Could you check a few things on this drawing? It's one solid part, dimensions in mm from its lowest x, y, z. A direction names the side the tool comes from. Give positions to 0.01 mm unless a question says otherwise; leave off trailing zeros. Order: outer loops, then holes, each group sorted by start corner. A loop starts at its lowest first (then second) coordinate and runs counter-clockwise, first axis right, second up. Notation, with made-up numbers: (4, -38) -> (26, -38) arc R20 cw to (26, -30) -> close; hole circle Ø1 at (-20, -31.75). An arc over 180 degrees is marked (long way). Use one line per item in the form item = value. Start each with the question number.
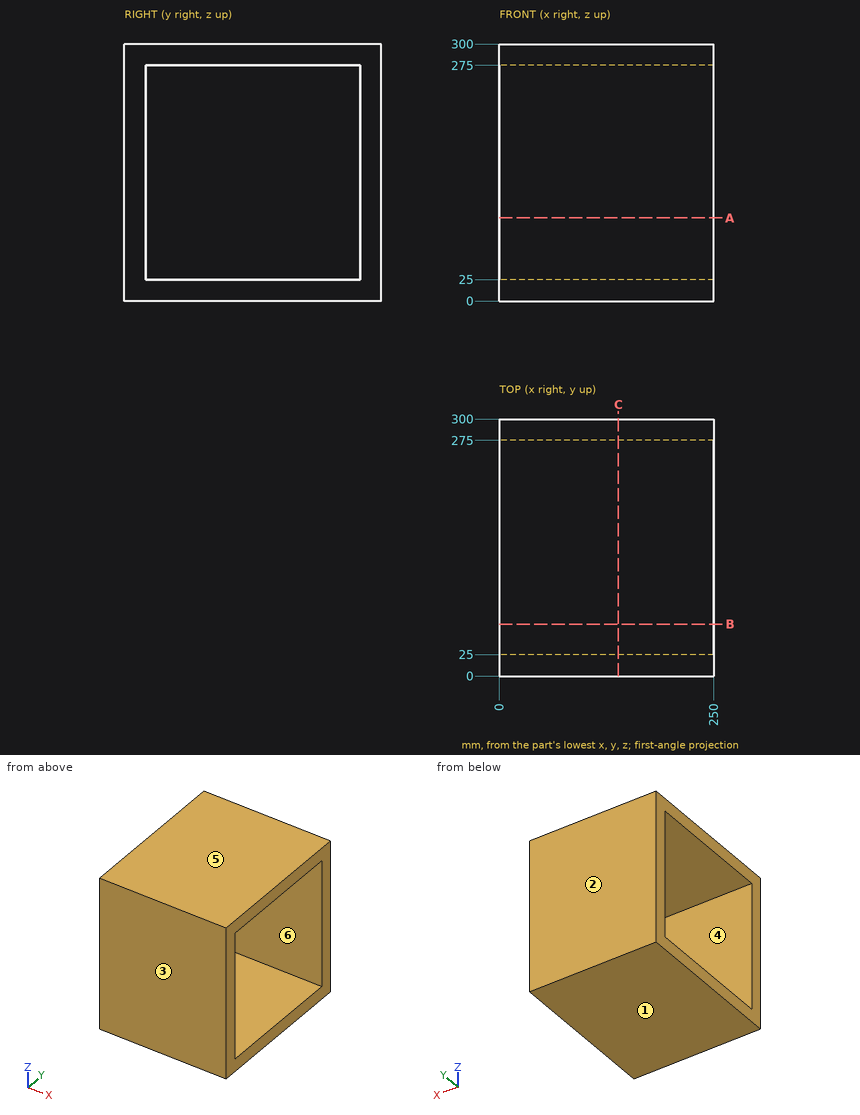
(1) Imagine slicing it at A-A (z = 97). Write out the boundary of the cut face in (x, y).
(2) Please list where this line runs through material, in increasing order: probe 1 along Z at (x, y) = (58.5, 240).
(3) I'm going to push a flat-ended pin straight in: pin 1 Ø3 at (x, z) = (95, 206) entering from -Y. Where does the tip first touch, or does it pass through?
(4) Which directions (+Z, -Z, +X, -X, +Y, -Y) give clear straight access to the entire face, cutting with the end or side of a thin tool? Please do the marked faces 5 and 6.
(5) We'd pull the mould along Y, two halves only. Please class the marked faces 1, 2, 3 and 4: pulls with the +Y half, pulls with the -Y half, needs draft (parallel to the pull), parting line crosses it, or undercut.
(6) Imagine slicing it at C-C (x = 139). Write out the boundary of the cut face in (y, z), plus the area to 3 significant figures.
Calculated:
q1.outline = (0, 0) -> (250, 0) -> (250, 25) -> (0, 25) -> close; (0, 275) -> (250, 275) -> (250, 300) -> (0, 300) -> close
q2.probe_1 = 0 to 25, 275 to 300
q3.pin_1 = 0
q4.face_5 = +Z, +X, -X, +Y, -Y
q4.face_6 = +X, -X
q5.face_1 = needs draft
q5.face_2 = pulls with the +Y half
q5.face_3 = pulls with the -Y half
q5.face_4 = undercut
q6.outline = (0, 0) -> (300, 0) -> (300, 300) -> (0, 300) -> close; hole (25, 25) -> (275, 25) -> (275, 275) -> (25, 275) -> close
q6.area = 27,500 mm2
